The drawing under review shows one solid part. Ordinate dimensions are in mm from its lowest x, y, z. A direction names the side the tool comes from. Round coordinates to 2 decimals unless told otherwise and drop trailing zeros. Write each loop counter-clockwise with the first axis right and the second up, starting at its lowest first coordinate (ties: lowest second). Pieces come first, ordered by that corner, then holes. Notation, with made-up numbers: M -23.75,-39.75 L 7.25,-39.75 A29 cw 7.25,-3.75 Z; hole C -9.75,63.25 d11. An arc over 180 degrees is marked long. One line per item, written item: value. Start each with the question number.
1) Take a section at A-A, the plane z = 9. Write out the cut boundary in (x, y).
2) Tool access review of the marked faces 1, 2 and 3: name each direction out of +Z, -Z, +X, -X, +Y, -Y from which nothing blocks a thin tool from reaching the whole face with its end or side.
3) For P1, Ø3, axis at x = 14, z = 2.5, coming from the +Y side; P2, Ø8, axis at x = 15.5, y = 5, coming from the +Z side, all flat-tipped, find the tip position at first contact; note any pin that passes through.
4) Take a section at C-C, the plane y = 13.25. Write out the cut boundary in (x, z), and give its area (3 significant figures).
5) Wall thickness on probe 1 along Z at (x, y) = (15.25, 9.5): over which ranges is the line inside the solid? List them lowest first.
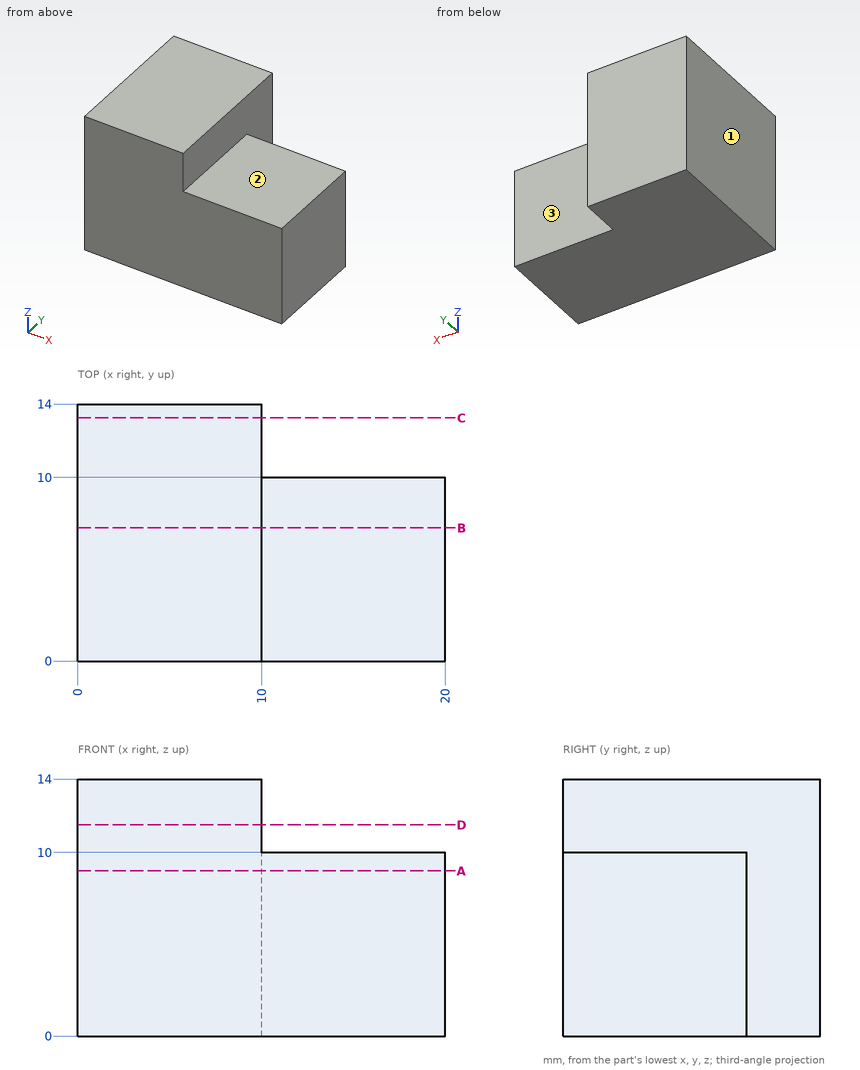
Checked values:
1. outline: M 0,0 L 20,0 L 20,10 L 10,10 L 10,14 L 0,14 Z
2. face 1: +Z, -Z, -X, +Y, -Y
2. face 2: +Z, +X, +Y, -Y
2. face 3: +Z, -Z, +X, +Y
3. P1: stops at y = 10
3. P2: stops at z = 10
4. outline: M 0,0 L 10,0 L 10,14 L 0,14 Z
4. area: 140 mm2
5. probe 1: z = 0 to 10
